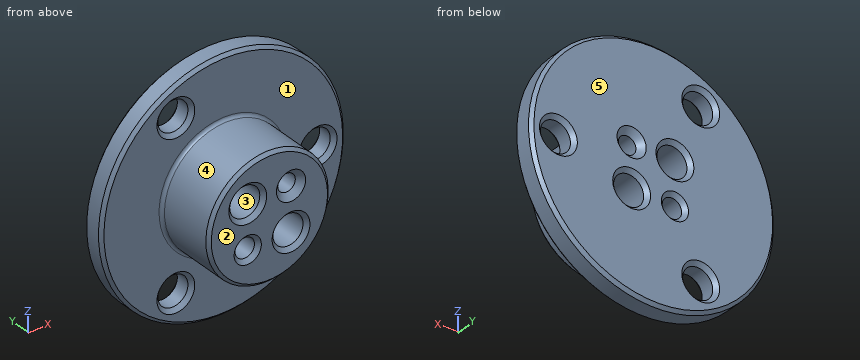
```python
from build123d import *

# Parameters (mm, degrees)
F_8_CLEARANCE_HOLE2_AT_2_COUNT = 2
F_8_CLEARANCE_HOLE2_AT_2_PITCH = 10
F_8_CLEARANCE_HOLE1_AT_2_COUNT = 2
F_8_CLEARANCE_HOLE1_AT_2_PITCH = 26.846787517
F_8_CLEARANCE_HOLE1_AT_3_COUNT = 2
F_8_CLEARANCE_HOLE1_AT_3_PITCH = 26.846787517
CHAMFER1_SIZE                  = 0.5
FILLET1_R                      = 0.5


with BuildPart() as part:
    # Sketch1 → Revolve1 (revolve)
    with BuildSketch(Plane(origin=(0, 0, 0), x_dir=(0, 0, -1), z_dir=(1, 0, 0)), mode=Mode.PRIVATE) as revolve1_sk:
        Polygon((0, 0), (0, 13.2432806), (20, 13.2432806), (20, 9.7432806), (10, 9.7432806), (10, 0), align=None)
    revolve(revolve1_sk.sketch.rotate(Axis((0, 0, 0), (0, -1, 0)), 180), axis=Axis((0, 0, 0), (0, -1, 0)))  # turned: the seam where the file's is

    # Sketch4 → #8 Clearance Hole2 (revolve, cut)
    with BuildSketch(Plane(origin=(3.535533906, 13.2432806, -3.535533906), x_dir=(0, 0, 1), z_dir=(1, 0, 0))):
        Polygon((0, 0), (0, 13.2432806), (3.09245, 13.2432806), (2.45745, 12.6082806), (2.45745, 0.635), (3.09245, 0), align=None)
    f_8_clearance_hole2 = revolve(axis=Axis((3.535533906, 19.5932806, -3.535533906), (0, -1, 0)), mode=Mode.SUBTRACT)

    # #8 Clearance Hole2 at 2: #8 Clearance Hole2 ×2
    with Locations(*[Vector(-0.707106781, 0, 0.707106781) * (i * F_8_CLEARANCE_HOLE2_AT_2_PITCH) for i in range(1, F_8_CLEARANCE_HOLE2_AT_2_COUNT)]):
        add(f_8_clearance_hole2, mode=Mode.SUBTRACT)

    # Sketch5 → 1/8 (0.125) Diameter Hole1 (revolve, cut)
    with BuildSketch(Plane(origin=(-3.535533906, 13.2432806, -3.535533906), x_dir=(0, 0, 1), z_dir=(1, 0, 0))):
        Polygon((0, 0), (0, 13.2432806), (2.2225, 13.2432806), (1.5875, 12.6082806), (1.5875, 0.635), (2.2225, 0), align=None)
    revolve(axis=Axis((-3.535533906, 19.5932806, -3.535533906), (0, -1, 0)), mode=Mode.SUBTRACT)

    # Sketch8 → #8 Clearance Hole1 (revolve, cut)
    with BuildSketch(Plane(origin=(-7.75, 13.2432806, -13.423393759), x_dir=(0, 0, 1), z_dir=(1, 0, 0))):
        Polygon((0, 0), (0, 3.5), (3.0861, 3.5), (2.45745, 2.87135), (2.45745, 0.635), (3.09245, 0), align=None)
    f_8_clearance_hole1 = revolve(axis=Axis((-7.75, 19.5932806, -13.423393759), (0, -1, 0)), mode=Mode.SUBTRACT)

    # #8 Clearance Hole1 at 2: #8 Clearance Hole1 ×2
    with Locations(*[Vector(0.866025404, 0, 0.5) * (i * F_8_CLEARANCE_HOLE1_AT_2_PITCH) for i in range(1, F_8_CLEARANCE_HOLE1_AT_2_COUNT)]):
        add(f_8_clearance_hole1, mode=Mode.SUBTRACT)

    # #8 Clearance Hole1 at 3: #8 Clearance Hole1 ×2
    with Locations(*[(0, 0, i * F_8_CLEARANCE_HOLE1_AT_3_PITCH) for i in range(1, F_8_CLEARANCE_HOLE1_AT_3_COUNT)]):
        add(f_8_clearance_hole1, mode=Mode.SUBTRACT)

    # Sketch10 → #6-40 Tapped Hole1 (revolve, cut)
    with BuildSketch(Plane(origin=(3.535533906, 13.2432806, 3.535533906), x_dir=(0, 0, 1), z_dir=(1, 0, 0))):
        Polygon((0, 0), (0, 13.2432806), (2.3876, 13.2432806), (1.4351, 12.2907806), (1.4351, 0.9525), (2.3876, 0), align=None)
    revolve(axis=Axis((3.535533906, 19.5932806, 3.535533906), (0, -1, 0)), mode=Mode.SUBTRACT)

    # Chamfer1
    chamfer1_edges = [part.edges().sort_by_distance(p)[0] for p in [
        (0, 0, -10),
        (0, 9.7432806, -20),
        (0, 13.2432806, -20),
    ]]
    chamfer(chamfer1_edges, length=CHAMFER1_SIZE)

    # Fillet1
    fillet1_edges = [part.edges().sort_by_distance(p)[0] for p in [
        (0, 9.7432806, -10),
    ]]
    fillet(fillet1_edges, radius=FILLET1_R)


solid = part.part
```
Check sheet for the modelled part. Datum: model origin and axes. Units: mm. Face numbers are marked on the shaded views. A direction names the side the tool comes from. Coordinates: 2 decimals unless noted, no trailing zeros. Write each loop counter-clockwise with the first axis right and the second up, starting at its lowest first coordinate (ties: lowest second). Pieces come first, ordered by that corner, then holes. Notation, with made-up numbers: M 67.25,34 L 123.25,34 A18 cw 123.25,53 Z; hole C -22.75,-40 d4. An arc over 180 degrees is marked long. Write item = value, one per line. Start each with the question number.
1. Sectioned sample at B-B (y = 4.5). Record the cut outline in (x, z) (1 decimal), then the cut area to 3 significant figures.
2. Sectioned sample at A-A (y = 11.5). State how many separate pieces and enclosed holes the cut face has, then the cut area to 3 significant figures.
3. Tool access check on the marked faces 1 and 2. Record the directions out of +Z, -Z, +X, -X, +Y, -Y that give a thin tool (end or side, any length) a straight path to the whole face; none if there is none.
4. Go/stop test with flat-tipped pins: pin 1 (5 mm diameter, centred on x = 10.5, y = 4, fed in from +Z); pin 2 (4 mm diameter, centred on x = -3.54, z = -3.54, fed in from -Y); pin 3 (3 mm diameter, centred on x = 13.5, y = 10.5, fed in from -Z). Record where each tip stops, or that it passes through.
5. Mould release check, pull along X, two halves, no side actions. Record for the marked faces 3, 4 and 5: pulls with the +X half, pulls with the -X half, needs draft (parallel to the pull), parting line crosses it, or undercut.
6. Thickness scan on probe 1 along X at (y, z) = (11.25, 0); probe 2 along X at (y, z) = (11.75, 4.5); probe 3 along Y at (x, z) = (-9, 10). Record the ranges inside material, lowest first.
The answers:
q1.outline = C 0,0 d20; hole C -3.5,3.5 d4.9; hole C -3.5,-3.5 d3.2; hole C 3.5,-3.5 d4.9; hole C 3.5,3.5 d2.9
q1.area = 262 mm²
q2.separate_pieces = 1
q2.enclosed_holes = 7
q2.area = 1,150 mm²
q3.face_1 = -Y
q3.face_2 = +Z, -Z, +X, -X, -Y
q4.pin_1 = 6
q4.pin_2 = 0.22
q4.pin_3 = -16
q5.face_3 = undercut
q5.face_4 = parting line crosses it
q5.face_5 = needs draft
q6.probe_1 = -20 to 13.04, 17.96 to 20
q6.probe_2 = -19.49 to -5.8, -1.28 to 2.47, 4.6 to 19.49
q6.probe_3 = 9.74 to 13.24
